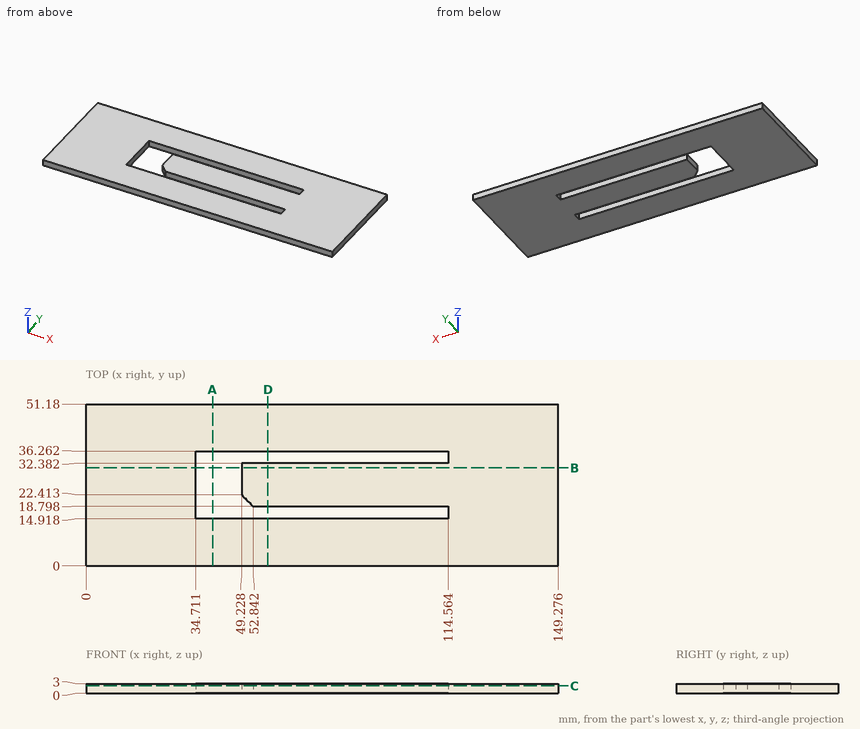
Design review of the part shown in the three views and the two pictorial views. Dimensions are in mm from the part's minimum x, y and z. Round coordinates to 2 decimals unless told otherwise and drop trailing zeros. Write each loop counter-clockwise with the first axis right and the second up, starting at its lowest first coordinate (ties: lowest second). Pieces come first, ordered by that corner, then holes. Notation, with made-up numbers: M 12.5,74.5 L 49.5,74.5 A10 cw 49.5,89.5 Z; hole C 70,65.25 d8. An arc over 180 degrees is marked long. Use a Markdown table: item, result. Add a question column.
Q1. We need section B-B, the plane y = 31. State the section outline as (x, z) points (1 decimal).
Q2. To check wall thickness, follow line 1 (Y direction, x = 103, z = 0.8); line 2 (X direction, y = 18, z = 2.15) (1 decimal); line 3 (X direction, y = 30, z = 1.8) (1 decimal). State the ranges of each line that lie inside material, in increasing order.
Q3. We need section A-A, the plane x = 40. State the section outline as (y, z) points.
Q4. We need section C-C, the plane z = 2.4. State the section outline as (x, y) points (1 decimal), plus the area to 3 significant figures.
Q5. We need section D-D, the plane x = 57.5. State the section outline as (y, z) points.
Findings below:
| question | item | result |
|---|---|---|
| 1 | outline | M 0,0 L 34.7,0 L 34.7,3 L 0,3 Z; M 49.2,0 L 149.3,0 L 149.3,3 L 49.2,3 Z |
| 2 | line 1 | y = 0 to 14.92, 18.8 to 32.38, 36.26 to 51.18 |
| 2 | line 2 | x = 0 to 34.7, 114.6 to 149.3 |
| 2 | line 3 | x = 0 to 34.7, 49.2 to 149.3 |
| 3 | outline | M 0,0 L 14.92,0 L 14.92,3 L 0,3 Z; M 36.26,0 L 51.18,0 L 51.18,3 L 36.26,3 Z |
| 4 | outline | M 0,0 L 149.3,0 L 149.3,51.2 L 0,51.2 Z; hole M 34.7,14.9 L 114.6,14.9 L 114.6,18.8 L 52.8,18.8 L 49.2,22.4 L 49.2,32.4 L 114.6,32.4 L 114.6,36.3 L 34.7,36.3 Z |
| 4 | area | 6,820 mm² |
| 5 | outline | M 0,0 L 14.92,0 L 14.92,3 L 0,3 Z; M 18.8,0 L 32.38,0 L 32.38,3 L 18.8,3 Z; M 36.26,0 L 51.18,0 L 51.18,3 L 36.26,3 Z |
